from build123d import *

# Parameters (mm, degrees)
F0_W     = 609.6
F0_H     = 381
F0_H_2   = 76.2
F1_DEPTH = 2286
F2_DEPTH = 114.3


with BuildPart() as f1:
    # F0 (on Top) → F1 (new body)
    with BuildSketch(Plane.XY):
        with Locations((0, 38.1)):
            Rectangle(F0_W, F0_H)
        with Locations((0, -190.5)):
            Rectangle(F0_W, F0_H_2)
    extrude(amount=F1_DEPTH)

    # F0 (on Top) → F2 (join)
    with BuildSketch(Plane.XY):
        with Locations((0, 38.1)):
            Rectangle(F0_W, F0_H)
    extrude(amount=-F2_DEPTH)


solid = f1.part
CAD build for the part. Positions are in the model's coordinates, mm. A direction names the side the tool comes from. Give positions to 0.01 mm unless a question says otherwise; leave off trailing zeros. Write each loop counter-clockwise with the first axis right and the second up, starting at its lowest first coordinate (ties: lowest second). Pieces come first, ordered by that corner, then holes. Notation, with made-up numbers: M 33,18 L 51,18 A24 cw 51,45 Z; hole C 41.5,64.5 d6. An arc over 180 degrees is marked long. Put each result on its own line as item: value. Start each with the question number.
(1) Flat gauge pin, fed straight in: pin 1 Ø23 at (x, y) = (-11, -202.5) entering from -Z. Where does the tip first touch, or does it go through?
(2) Mould opens along X. For faces 1 (the face through (-304.8, -3, 1103)), 2 (the face through (-4, -228.6, 1127)), 3 (the face through (304.8, -3, 1103)) say: +X half, -X half, draft (parallel to the pull), parting line (faces both ways), or undercut.
(3) Which spindle directions (+Z, -Z, +X, -X, +Y, -Y) get a long thin tool onto all of the face, cutting with end or side? Do faces 4 (the face through (-4, -152.4, -56)), 5 (the face through (-4, 228.6, 1103)). Say none if no direction does.
(4) Probe L1, parallel to Z at x = -8.5, y = -200.5. List the from-to ranges inside material, lowest first.
(5) Band-saw the part on A-A, the plane y = -177. Write the cut outline in (x, z).
Response values:
1. pin 1: stops at z = 0
2. face 1: -X half
2. face 2: draft
2. face 3: +X half
3. face 4: -Z, +X, -X, -Y
3. face 5: +Z, -Z, +X, -X, +Y
4. L1: z = 0 to 2286
5. outline: M -304.8,0 L 304.8,0 L 304.8,2286 L -304.8,2286 Z
